Input: part model. Units: mm. Frame: model coordinates. Face numbers are marked on the shaded views. A direction names the side the tool comes from. Round coordinates to 2 decimals unless told otherwise and drop trailing zeros. Loops run counter-clockwise (first coordinate to the right, second up) from the corner with the lowest first, then second, coordinate; pieces in that order, holes last. Notation, with made-up numbers: (34, 62.5) - (62, 62.5) arc R9 cw to (62, 77.5) - close; hole circle Ø7 at (-26, -28). An arc over 180 degrees is marked (long way). One line per question, with ' | ' between items. Start each with the question number.
Item 1: Section A-A, the plane z = 6. Return loops of the section in (x, y), plus the area to 3 significant figures.
Item 2: Set-up query: the marked faces 1, 2 and 3. Return all of +Z, -Z, +X, -X, +Y, -Y with unobstructed straight access to the full face (end or side cutting, diameter ignored); none if empty.
Item 3: First-contact query: pin 1 (3 mm diameter, centred on x = 15.5, z = 0, fed in from -Y); pin 2 (8 mm diameter, centred on x = -1.5, z = -4, fed in from -Y); pin 3 (0.5 mm diameter, centred on x = 4.5, y = 1, fed in from +Z); pin 4 (10 mm diameter, centred on x = 4.5, z = 3.5, fed in from +Y). Flat tips, straight axial feed; report the tip coordinate or a pass-through.
Item 4: Section C-C, the plane y = -0.5. Return loops of the section in (x, z), plus the area to 3 significant figures.
Item 5: Section D-D, the plane x = -2. Return loops of the section in (y, z).
Item 6: Material intervals for line 1 along Y through (x, z) = (-3, -10.5); line 2 along X through (y, z) = (1.5, -3.5); line 3 along X through (y, z) = (-1.5, -3.75), sorted ascending.
Item 7: Section B-B, the plane x = 2. Return loops of the section in (y, z), plus the area to 3 significant figures.
```python
from build123d import *

# Parameters (mm, degrees)
F0_W     = 25.4
F0_H     = 25.4
F0_R     = 1.190625
F0_W_2   = 8.73125
F0_H_2   = 8.73125
F0_R_2   = 3.96875
F1_DEPTH = 1.016
F2_DEPTH = 1.5875
F3_DEPTH = 4.7625
F4_R     = 1.524
F5_W     = 5.55625
F5_H     = 21.283928
F6_DEPTH = 2.95275
F7_W     = 0.254
F7_H     = 15.875
F8_DEPTH = 6.35


with BuildPart() as f1:
    # F0 (on Front) → F1 (new body)
    with BuildSketch(Plane.XZ):
        with Locations((0.840441, -0.954741)):
            Rectangle(F0_W, F0_H)
        with Locations((-9.875184, -11.670366)):
            Circle(F0_R, mode=Mode.SUBTRACT)
        with Locations((2.824816, -11.670366)):
            Circle(F0_R, mode=Mode.SUBTRACT)
        with Locations((2.824816, -0.954741)):
            Rectangle(F0_W_2, F0_H_2, mode=Mode.SUBTRACT)
        with Locations((-9.875184, 9.760884)):
            Circle(F0_R, mode=Mode.SUBTRACT)
        with Locations((2.824816, 9.760884)):
            Circle(F0_R, mode=Mode.SUBTRACT)
        with Locations((2.824816, -0.954741)):
            Rectangle(F0_W_2, F0_H_2)
        with Locations((2.824816, -0.954741)):
            Circle(F0_R_2, mode=Mode.SUBTRACT)
        with Locations((2.824816, -0.954741)):
            Circle(F0_R_2)
    extrude(amount=F1_DEPTH)

    # F0 (on Front) → F2 (join)
    with BuildSketch(Plane.XZ):
        with Locations((2.824816, -0.954741)):
            Rectangle(F0_W_2, F0_H_2)
        with Locations((2.824816, -0.954741)):
            Circle(F0_R_2, mode=Mode.SUBTRACT)
        with Locations((2.824816, -0.954741)):
            Circle(F0_R_2)
    extrude(amount=-F2_DEPTH)

    # F0 (on Front) → F3 (join)
    with BuildSketch(Plane.XZ):
        with Locations((2.824816, -0.954741)):
            Circle(F0_R_2)
    extrude(amount=-F3_DEPTH)

    # F4
    f4_edges = [f1.edges().sort_by_distance(p)[0] for p in [
        (-11.859559, -0.508, 11.745259),
        (-11.859559, -0.508, -13.654741),
        (13.540441, -0.508, -13.654741),
        (13.540441, -0.508, 11.745259),
    ]]
    fillet(f4_edges, radius=F4_R)

    # F5 (on face) → F6 (join)
    with BuildSketch(Plane.XZ.offset(1.016)):
        with Locations((10.762316, -0.954741)):
            Rectangle(F5_W, F5_H)
    extrude(amount=F6_DEPTH)

    # F7 (on face) → F8 (join)
    with BuildSketch(Plane.YZ.offset(13.540441)):
        with Locations((-1.905, 0)):
            Rectangle(F7_W, F7_H)
    extrude(amount=F8_DEPTH)


solid = f1.part
```
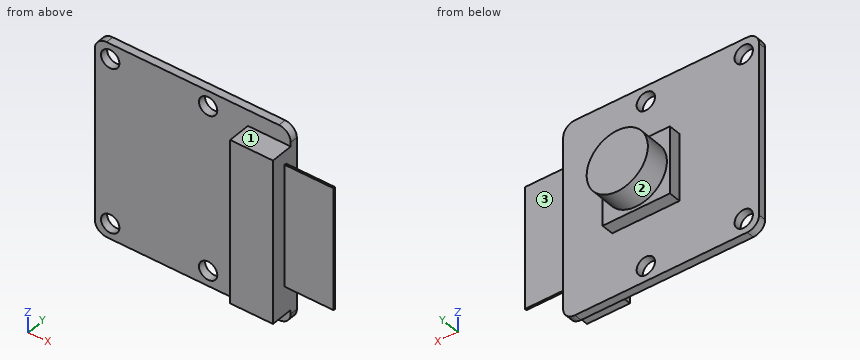
Return value:
1) outline: (-11.86, -1.02) - (7.98, -1.02) - (7.98, -3.97) - (13.54, -3.97) - (13.54, -2.03) - (19.89, -2.03) - (19.89, -1.78) - (13.54, -1.78) - (13.54, 0) - (-11.86, 0) - close | area: 43.8 mm2
2) face 1: +Z, +X, -X, -Y | face 2: +Y | face 3: +Z, -Z, +X, +Y
3) pin 1: y = -2.03 | pin 2: y = -1.02 | pin 3: z = 3.41 | pin 4: y = 4.76
4) outline: (-11.86, -12.13) arc R1.52 ccw to (-10.34, -13.65) - (12.02, -13.65) arc R1.52 ccw to (13.54, -12.13) - (13.54, 10.22) arc R1.52 ccw to (12.02, 11.75) - (-10.34, 11.75) arc R1.52 ccw to (-11.86, 10.22) - close; hole circle Ø2.38 at (-9.88, -11.67); hole circle Ø2.38 at (-9.88, 9.76); hole circle Ø2.38 at (2.82, -11.67); hole circle Ø2.38 at (2.82, 9.76) | area: 625 mm2
5) outline: (-1.02, -13.65) - (0, -13.65) - (0, 11.75) - (-1.02, 11.75) - close
6) line 1: -1.02 to 0 | line 2: -1.54 to 7.19 | line 3: 7.98 to 13.54
7) outline: (-1.02, -13.65) - (0, -13.65) - (0, -12.53) - (-1.02, -12.53) - close; (-1.02, -10.81) - (0, -10.81) - (0, -5.32) - (1.59, -5.32) - (1.59, -4.84) - (4.76, -4.84) - (4.76, 2.93) - (1.59, 2.93) - (1.59, 3.41) - (0, 3.41) - (0, 8.9) - (-1.02, 8.9) - close; (-1.02, 10.62) - (0, 10.62) - (0, 11.75) - (-1.02, 11.75) - close | area: 60.8 mm2
